from build123d import *

# Parameters (mm, degrees)
F1_DEPTH  = 25.4
F2_R      = 8.894978
F3_DEPTH  = 12.7
F4_DEPTH  = 25.4
F5_R      = 7.065357
F6_DEPTH  = 19.05
F7_W      = 13.161447
F7_H      = 7.129116
F8_DEPTH  = 25.401
F9_R      = 6.35
F10_DEPTH = 25.401
F11_R     = 5.08
F12_R     = 5.08


with BuildPart() as f1:
    # F0 (on Front) → F1 (new body)
    with BuildSketch(Plane.XZ):
        Polygon((-8.872092, 41.864544), (-39.002884, 50.96459), (-39.002884, 10.889949), (-8.872092, 9.806205), align=None)
    extrude(amount=F1_DEPTH)

    # F2 (on face) → F3 (join)
    with BuildSketch(Plane.YZ.offset(-8.872092)):
        with Locations((-12.7, 24.323635)):
            Circle(F2_R)
    extrude(amount=-F3_DEPTH)

    # F2 (on face) → F4 (cut)
    with BuildSketch(Plane.YZ.offset(-8.872092)):
        with Locations((-12.7, 24.323635)):
            Circle(F2_R)
    extrude(amount=-F4_DEPTH, mode=Mode.SUBTRACT)

    # F5 (on face) → F6 (join)
    with BuildSketch(Plane(origin=(0.340791, 0, 9.474836), x_dir=(0.999354, 0, -0.035945), z_dir=(-0.035945, 0, -0.999354))):
        with Locations((-24.293978, 12.492171)):
            Circle(F5_R)
    extrude(amount=F6_DEPTH)

    # F7 (on Front) → F8 (cut, through all)
    with BuildSketch(Plane.XZ):
        with Locations((-27.840523, 0.226574)):
            Rectangle(F7_W, F7_H)
    extrude(amount=F8_DEPTH, mode=Mode.SUBTRACT)

    # F9 (on face) → F10 (cut, through all)
    with BuildSketch(Plane(origin=(0, 0, 0), x_dir=(-1, 0, 0), z_dir=(0, 1, 0))):
        with Locations((8.872092, 25.835374)):
            Circle(F9_R)
    extrude(amount=-F10_DEPTH, mode=Mode.SUBTRACT)

    # F11
    f11_edges = [f1.edges().sort_by_distance(p)[0] for p in [
        (-39.002884, 0, 30.92727),
    ]]
    fillet(f11_edges, radius=F11_R)

    # F12
    f12_edges = [f1.edges().sort_by_distance(p)[0] for p in [
        (-39.002884, -25.4, 30.92727),
    ]]
    fillet(f12_edges, radius=F12_R)


solid = f1.part
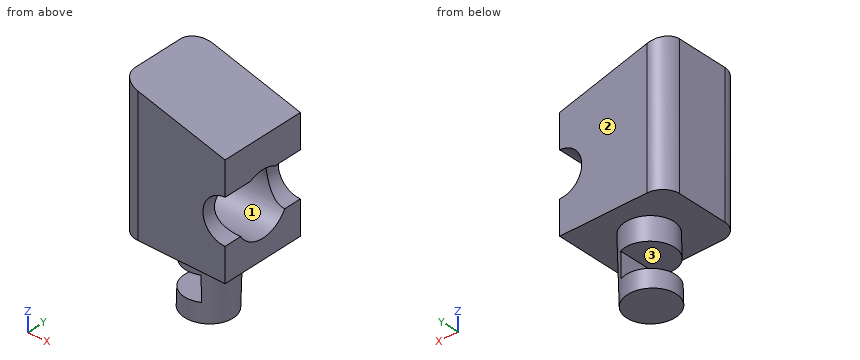
Geometry: final body of the model. Coordinates: model frame, mm. Face numbers are marked on the shaded views. A direction names the side the tool comes from. Give positions to 0.01 mm unless a question says otherwise; leave off trailing zeros. Write each loop counter-clockwise with the first axis right and the second up, starting at its lowest first coordinate (ties: lowest second). Pieces come first, ordered by that corner, then holes. Notation, with made-up numbers: M 9.25,3.5 L 56.25,3.5 A24 cw 56.25,13.5 Z; hole C 34,9.5 d11. An arc over 180 degrees is marked long. Answer in a Markdown table with one row per item. Add a question column.
(1) Ray query, line 1 (Z direction, x = -25.25, y = -12.7); line 2 (Z direction, x = -25.5, y = -12.7); line 3 (Z direction, x = -15, y = -12.7). Return the intervals inside material, ascending.
(2) First-contact query: pin 1 (3 mm diameter, centred on x = -28, y = -12.5, fed in from +Z); pin 2 (12 mm diameter, centred on x = -16, y = -17.5, fed in from -Z); pin 3 (12 mm diameter, centred on x = -26.5, y = -14, fed in from +Z); pin 4 (3.5 mm diameter, centred on y = -9.5, z = 1.5, fed in from -X). Flat tips, straight axial feed; report the tip coordinate or a pass-through.
(3) Reachability of the marked faces 1, 2 and 3 from +Z, -Z, +X, -X, +Y, -Y: full face, straight path, thin tool, end or side. Return the list, or none.
(4) Section B-B on y = -11.5. Return loops of the section in (x, z), and give its area (3 significant figures).
(5) Section A-A on z = 16.5. Return loops of the section in (x, y).
(6) Section C-C on x = -36.5. Return loops of the section in (y, z).
Result set:
| question | item | result |
|---|---|---|
| 1 | line 1 | z = -8.67 to -3.34, 3.79 to 15.43, 33.22 to 46.81 |
| 1 | line 2 | z = -8.66 to -3.34, 3.79 to 15.43, 33.22 to 46.89 |
| 1 | line 3 | z = 10.03 to 15.43, 33.22 to 43.72 |
| 2 | pin 1 | stops at z = 48.09 |
| 2 | pin 2 | stops at z = -8.94 |
| 2 | pin 3 | stops at z = 49 |
| 2 | pin 4 | stops at x = -21.26 |
| 3 | face 1 | +X |
| 3 | face 2 | +Z, -Z, +X, -X, +Y |
| 3 | face 3 | -X, +Y, -Y |
| 4 | outline | M -39,10.89 L -30.93,10.6 L -31.17,3.79 L -21.26,3.79 L -21.26,-3.34 L -31.43,-3.34 L -31.61,-8.44 L -17.63,-8.94 L -16.95,10.1 L -8.87,9.81 L -8.87,15.51 L -34.27,15.51 L -34.27,33.14 L -8.87,33.14 L -8.87,41.86 L -39,50.96 Z |
| 4 | area | 834 mm^2 |
| 5 | outline | M -39,-20.32 A5.08 ccw -33.92,-25.4 L -8.87,-25.4 L -8.87,-16.93 L -34.27,-16.93 L -34.27,-8.47 L -8.87,-8.47 L -8.87,0 L -33.92,0 A5.08 ccw -39,-5.08 Z |
| 6 | outline | M -24.7,10.8 L -0.7,10.8 L -0.7,50.21 L -24.7,50.21 Z |
